Geometry check sheet. Reference: the model listing, model coordinates, mm. Face numbers are marked on the shaded views. A direction names the side the tool comes from. Round coordinates to 2 decimals unless told otherwise and drop trailing zeros. Write each loop counter-clockwise with the first axis right and the second up, starting at its lowest first coordinate (ties: lowest second). Pieces come first, ordered by that corner, then holes.
Item 1: Cross-section at D-D (x = 3.25). Enter the section's corners in (y, z), then the cut area to 3 significant figures.
Item 2: Draft check along Z on the marked faces 1, 2 and 3. Enter one of: pulls with the +Z half, pulls with the -Z half, needs draft (parallel to the pull), parting line crosses it, or undercut.
Item 3: Depth check by flat-ended pin: P1, Ø8, axis at x = 4, y = 0, coming from the +Z side; P2, Ø4, axis at x = 3.5, y = -5, coming from the +Z side; P3, Ø3, axis at y = 2, z = 19, coming from the -X side; P4, Ø5, axis at y = 3.5, z = 20, coming from the +X side. Enter the tip coordinate at first touch or a pass-through.
Item 4: Cross-section at B-B (y = -0.75). Enter the section's corners in (x, z) (3 decimals), then the cut area to 3 significant figures.
Item 5: Access from +Z, -Z, +X, -X, +Y, -Y to the whole of each face (thin tool, end or side, straight path). Record for the marked faces 4 and 5.
Item 6: Cross-section at A-A (x = 0). Enter the section's corners in (y, z) (3 decimals).
Item 7: Scan lines: probe 1 along Z at (x, y) = (-4, -1); probe 2 along Z at (x, y) = (-2.75, 5.25); probe 3 along Y at (x, z) = (-2, 11.5). Record each from-to range of solid material in increasing order.
Item 8: Cross-section at C-C (z = 8). Enter the section's corners in (x, y) (3 decimals).
from build123d import *

# Parameters (mm, degrees)
SKETCH1_R           = 8
BOSS_EXTRUDE1_DEPTH = 3
SKETCH2_R           = 4.575
BOSS_EXTRUDE2_DEPTH = 14
SKETCH3_R           = 2.5
BOSS_EXTRUDE3_DEPTH = 10
SKETCH4_R           = 1.325
CUT_EXTRUDE1_DEPTH  = 7.5


with BuildPart() as part:
    # Sketch1 → Boss-Extrude1 (new body)
    with BuildSketch(Plane.XY):
        Circle(SKETCH1_R)
    extrude(amount=BOSS_EXTRUDE1_DEPTH)

    # Sketch2 → Boss-Extrude2 (add)
    with BuildSketch(Plane.XY.offset(3)):
        Circle(SKETCH2_R)
    extrude(amount=BOSS_EXTRUDE2_DEPTH)

    # Sketch3 → Boss-Extrude3 (add)
    with BuildSketch(Plane.XY.offset(17)):
        Circle(SKETCH3_R)
    extrude(amount=BOSS_EXTRUDE3_DEPTH)

    # Sketch4 → Cut-Extrude1 (cut, symmetric)
    with BuildSketch(Plane(origin=(0, 0, 0), x_dir=(1, 0, 0), z_dir=(0, 1, 0))):
        with Locations((0.425, -13.99354762)):
            Circle(SKETCH4_R)
    extrude(amount=CUT_EXTRUDE1_DEPTH, both=True, mode=Mode.SUBTRACT)


solid = part.part
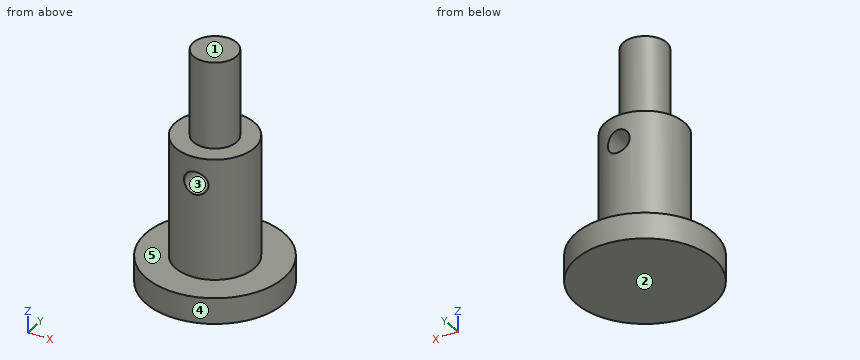
Resolved:
1. outline: (-7.31, 0) - (7.31, 0) - (7.31, 3) - (3.22, 3) - (3.22, 17) - (-3.22, 17) - (-3.22, 3) - (-7.31, 3) - close
1. area: 134 mm2
2. face 1: pulls with the +Z half
2. face 2: pulls with the -Z half
2. face 3: undercut
3. P1: stops at z = 27
3. P2: stops at z = 17
3. P3: stops at x = -2.45
3. P4: stops at x = 2.29
4. outline: (-7.965, 0) - (7.965, 0) - (7.965, 3) - (4.513, 3) - (4.513, 17) - (2.385, 17) - (2.385, 27) - (-2.385, 27) - (-2.385, 17) - (-4.513, 17) - (-4.513, 3) - (-7.965, 3) - close; hole circle Ø2.65 at (0.425, 13.994)
4. area: 216 mm2
5. face 4: +Z, -Z
5. face 5: +Z
6. outline: (-8, 0) - (8, 0) - (8, 3) - (4.575, 3) - (4.575, 12.739) - (-4.575, 12.739) - (-4.575, 3) - (-8, 3) - close; (-4.575, 15.249) - (4.575, 15.249) - (4.575, 17) - (2.5, 17) - (2.5, 27) - (-2.5, 27) - (-2.5, 17) - (-4.575, 17) - close
7. probe 1: z = 0 to 17
7. probe 2: z = 0 to 3
7. probe 3: y = -4.11 to 4.11
8. outline: circle Ø9.15 at (0, 0)
